Geometry check sheet. Reference: drawing and pictorial views, mm from the part's lowest x, y, z. Give positions to 0.01 mm unless a question says otherwise; leave off trailing zeros. Order: outer loops, then holes, each group sorted by start corner. A loop starts at its lowest first (then second) coordinate and runs counter-clockwise, first axis right, second up. Notation, with made-up numbers: (24.5, 11.25) - (40.5, 11.25) arc R21 cw to (40.5, 32.25) - close; hole circle Ø1 at (62, 0). An arc over 180 degrees is marked (long way). Answer in a Markdown table with one row per item.
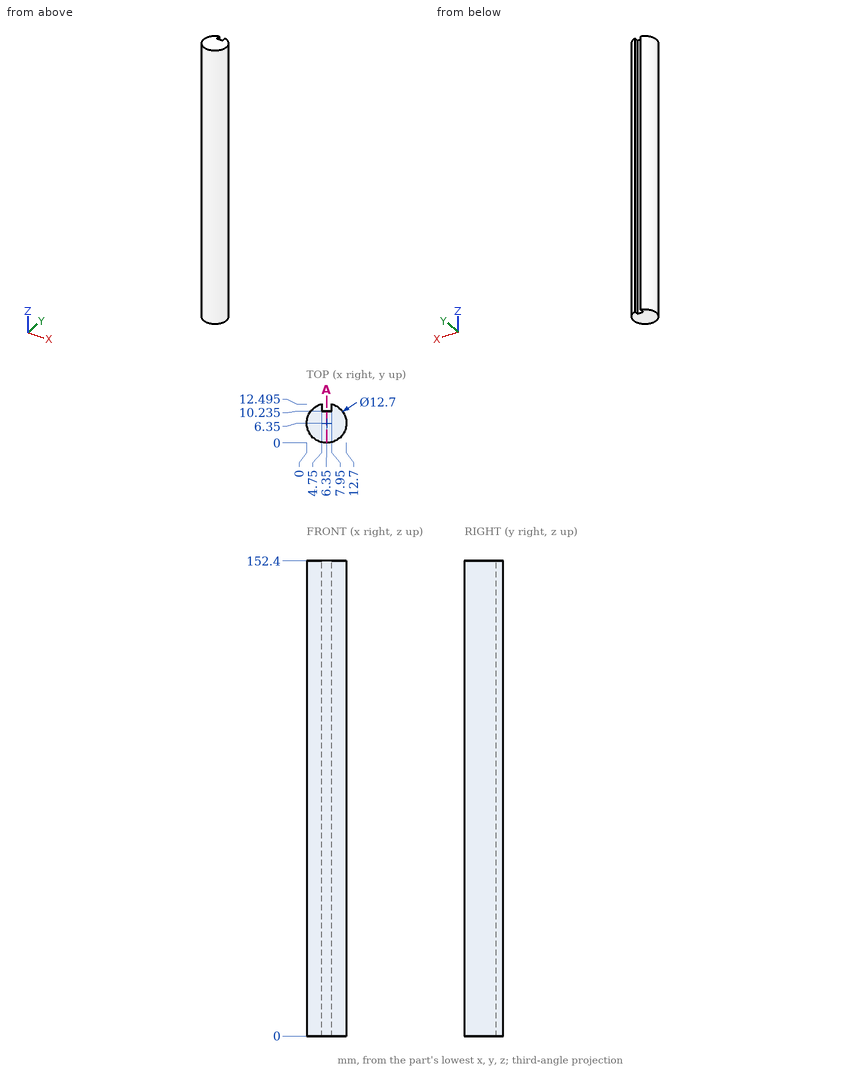
(1) Gauge pin test, flat ends, axial feed: P1, Ø1.1, axis at y = 11, z = 85, coming from the +X side; P2, Ø1.5, axis at x = 5, z = 118, coming from the +Y side (1 decimal); P3, Ø1.5, axis at x = 2.5, z = 41.5, coming from the +Y side; P4, Ø2, axis at x = 7, y = 6.5, coming from the -Z side. Record the tip position at first contact, or that the pin passes through.
Geometry says:
| item | result |
|---|---|
| P1 | x = 11.2 |
| P2 | y = 12.5 |
| P3 | y = 11.89 |
| P4 | z = 0 |
(2) Cross-section at A-A, the plane x = 6.35. Record the cut outline in (y, z) (1 decimal).
Geometry says:
| item | result |
|---|---|
| outline | (0, 0) - (10.2, 0) - (10.2, 152.4) - (0, 152.4) - close |
(3) Thickness scan on L1, parallel to Y at x = 6.25, z = 109 (1 decimal); L2, parallel to X at y = 1.75, z = 33.5 (1 decimal); L3, parallel to Y at x = 8.25, z = 60.5. Record the ranges inside material, lowest first.
Geometry says:
| item | result |
|---|---|
| L1 | 0 to 10.2 |
| L2 | 2 to 10.7 |
| L3 | 0.29 to 12.41 |
